Design review of the part built by this model. Coordinates are the model's own, in mm. A direction names the side the tool comes from. Give positions to 0.01 mm unless a question says otherwise; leave off trailing zeros. Write each loop counter-clockwise with the first axis right and the second up, starting at its lowest first coordinate (ties: lowest second). Pieces come first, ordered by that corner, then holes. Notation, with made-up numbers: M 89.25,6 L 126.25,6 A5 ccw 126.25,13 Z; hole C 76.25,8 d3. An arc over 180 degrees is marked long. Answer in a Markdown table with one row per item.
```python
from build123d import *

# Parameters (mm, degrees)
BOSS_EXTRUDE1_DEPTH = 203.2
SKETCH2_R           = 6.35
BOSS_EXTRUDE2_DEPTH = 12.7


with BuildPart() as part:
    # Sketch1 → Boss-Extrude1 (new body)
    with BuildSketch(Plane(origin=(0, 0, 0), x_dir=(0, 0, -1), z_dir=(1, 0, 0))):
        Polygon((6.72189532, -2.929070951), (5.897597513, 4.356796634), (-0.824297807, 7.285867584), (-6.72189532, 2.929070951), (-5.897597513, -4.356796634), (0.824297807, -7.285867584), align=None)
    extrude(amount=BOSS_EXTRUDE1_DEPTH)

    # Sketch2 → Boss-Extrude2 (add)
    with BuildSketch(Plane.ZY):
        Circle(SKETCH2_R)
    extrude(amount=BOSS_EXTRUDE2_DEPTH)


solid = part.part
```
1) To check wall thickness, follow probe 1 along Y at (x, z) = (154, -4.75); probe 2 along Z at (x, y) = (118, 3.75); probe 3 along Z at (x, y) = (46, 4.75). State the ranges of each line that lie inside material, in increasing order. Write a range as [from, to].
Geometry says:
| item | result |
|---|---|
| probe 1 | [-4.39, 4.86] |
| probe 2 | [-5.97, 5.61] |
| probe 3 | [-5, 4.26] |
2) Insertion check: P1, Ø1.7, axis at y = -6.5, z = -1, coming from the -X side; P2, Ø1, axis at x = 82, y = -1.5, coming from the +Z side; P3, Ø5, axis at x = 144.5, z = -1.5, coming from the -Y side; P4, Ø5, axis at x = 146.5, z = -2, coming from the +Y side. Each pin has a flat end and moves straight along its axis. Give the tip position at first contact, or say it passes through.
Geometry says:
| item | result |
|---|---|
| P1 | x = -12.7 |
| P2 | z = 6.28 |
| P3 | y = -7.29 |
| P4 | y = 7.14 |
3) Add section A-A (x = 87). Write out the cut boundary in (y, z).
Geometry says:
| item | result |
|---|---|
| outline | M -7.29,-0.82 L -2.93,-6.72 L 4.36,-5.9 L 7.29,0.82 L 2.93,6.72 L -4.36,5.9 Z |
4) For faces 1 (the face through (0, 3.8, -5.3)), 2 (the face through (0, -3.8, 5.3)), 3 (the face through (-6.26, -6.2, -1.38)), list the 3-axis set-ups (+Z, -Z, +X, -X, +Y, -Y) from which the entire face can be reached by the end or side of a thin tool; tool diameter is ignored.
Geometry says:
| item | result |
|---|---|
| face 1 | -Z, -X, +Y |
| face 2 | +Z, -X, -Y |
| face 3 | -X |
